Input: part model. Units: mm. Frame: model coordinates. Coordinates: 2 decimals unless noted, no trailing zeros. Order: outer loops, then holes, each group sorted by start corner. A loop starts at its lowest first (then second) coordinate and runs counter-clockwise, first axis right, second up. Notation, with made-up numbers: M -3.75,25.5 L 36.25,25.5 A20 cw 36.25,40.5 Z; hole C -10.5,9 d9. An arc over 180 degrees is marked long. One line per item, written item: value.
```python
from build123d import *

# Parameters (mm, degrees)
SKETCH2_W                = 22
SKETCH2_H                = 5
BOSS_EXTRUDE2_DEPTH      = 7.5
SKETCH16_W               = 0.596885676
SKETCH16_H               = 0.19726192
BOSS_EXTRUDE6_DEPTH      = 0.5
SKETCH17_W               = 0.596885676
SKETCH17_H               = 0.196118077
BOSS_EXTRUDE7_DEPTH      = 7.4
LPATTERN2_COUNT          = 10
LPATTERN2_PITCH          = 2.2
MIRROR1_COPY_1_SKETCH_W  = 0.596885676
MIRROR1_COPY_1_SKETCH_H  = 0.19726192
MIRROR1_COPY_1_DEPTH     = 0.5
MIRROR1_COPY_2_SKETCH_W  = 0.596885676
MIRROR1_COPY_2_SKETCH_H  = 0.19726192
MIRROR1_COPY_2_DEPTH     = 0.5
MIRROR1_COPY_3_SKETCH_W  = 0.596885676
MIRROR1_COPY_3_SKETCH_H  = 0.19726192
MIRROR1_COPY_3_DEPTH     = 0.5
MIRROR1_COPY_4_SKETCH_W  = 0.596885676
MIRROR1_COPY_4_SKETCH_H  = 0.19726192
MIRROR1_COPY_4_DEPTH     = 0.5
MIRROR1_COPY_5_SKETCH_W  = 0.596885676
MIRROR1_COPY_5_SKETCH_H  = 0.19726192
MIRROR1_COPY_5_DEPTH     = 0.5
MIRROR1_COPY_6_SKETCH_W  = 0.596885676
MIRROR1_COPY_6_SKETCH_H  = 0.19726192
MIRROR1_COPY_6_DEPTH     = 0.5
MIRROR1_COPY_7_SKETCH_W  = 0.596885676
MIRROR1_COPY_7_SKETCH_H  = 0.19726192
MIRROR1_COPY_7_DEPTH     = 0.5
MIRROR1_COPY_8_SKETCH_W  = 0.596885676
MIRROR1_COPY_8_SKETCH_H  = 0.19726192
MIRROR1_COPY_8_DEPTH     = 0.5
MIRROR1_COPY_9_SKETCH_W  = 0.596885676
MIRROR1_COPY_9_SKETCH_H  = 0.19726192
MIRROR1_COPY_9_DEPTH     = 0.5
MIRROR1_COPY_10_SKETCH_W = 0.596885676
MIRROR1_COPY_10_SKETCH_H = 0.196118077
MIRROR1_COPY_10_DEPTH    = 7.4
MIRROR1_COPY_11_SKETCH_W = 0.596885676
MIRROR1_COPY_11_SKETCH_H = 0.196118077
MIRROR1_COPY_11_DEPTH    = 7.4
MIRROR1_COPY_12_SKETCH_W = 0.596885676
MIRROR1_COPY_12_SKETCH_H = 0.196118077
MIRROR1_COPY_12_DEPTH    = 7.4
MIRROR1_COPY_13_SKETCH_W = 0.596885676
MIRROR1_COPY_13_SKETCH_H = 0.196118077
MIRROR1_COPY_13_DEPTH    = 7.4
MIRROR1_COPY_14_SKETCH_W = 0.596885676
MIRROR1_COPY_14_SKETCH_H = 0.196118077
MIRROR1_COPY_14_DEPTH    = 7.4
MIRROR1_COPY_15_SKETCH_W = 0.596885676
MIRROR1_COPY_15_SKETCH_H = 0.196118077
MIRROR1_COPY_15_DEPTH    = 7.4
MIRROR1_COPY_16_SKETCH_W = 0.596885676
MIRROR1_COPY_16_SKETCH_H = 0.196118077
MIRROR1_COPY_16_DEPTH    = 7.4
MIRROR1_COPY_17_SKETCH_W = 0.596885676
MIRROR1_COPY_17_SKETCH_H = 0.196118077
MIRROR1_COPY_17_DEPTH    = 7.4
MIRROR1_COPY_18_SKETCH_W = 0.596885676
MIRROR1_COPY_18_SKETCH_H = 0.196118077
MIRROR1_COPY_18_DEPTH    = 7.4


with BuildPart() as part:
    # Sketch2 → Boss-Extrude2 (new body)
    with BuildSketch(Plane(origin=(0, 5.922936542, 0), x_dir=(1, 0, 0), z_dir=(0, 0, 1))):
        with Locations((11, 2.5)):
            Rectangle(SKETCH2_W, SKETCH2_H)
    extrude(amount=BOSS_EXTRUDE2_DEPTH)

    # Sketch16 → Boss-Extrude6 (add)
    with BuildSketch(Plane.XY):
        with Locations((21, 8.422)):
            Rectangle(SKETCH16_W, SKETCH16_H)
    boss_extrude6 = extrude(amount=-BOSS_EXTRUDE6_DEPTH)

    # Sketch17 → Boss-Extrude7 (add)
    with BuildSketch(Plane.XZ.offset(-8.32336904)):
        with Locations((21, -0.401940962)):
            Rectangle(SKETCH17_W, SKETCH17_H)
    boss_extrude7 = extrude(amount=BOSS_EXTRUDE7_DEPTH)

    # LPattern2: Boss-Extrude6, Boss-Extrude7 ×10
    with Locations(*[(-i * LPATTERN2_PITCH, 0, 0) for i in range(1, LPATTERN2_COUNT)]):
        add(boss_extrude6)
        add(boss_extrude7)

    # Mirror1: Boss-Extrude6, Boss-Extrude7 across plane
    add(boss_extrude6.mirror(Plane(origin=(0, 0, 3.75), x_dir=(1, 0, 0), z_dir=(0, 0, -1))))
    add(boss_extrude7.mirror(Plane(origin=(0, 0, 3.75), x_dir=(1, 0, 0), z_dir=(0, 0, -1))))

    # Mirror1 copy 1 sketch → Mirror1 copy 1 (add)
    with BuildSketch(Plane(origin=(-2.2, 0, 7.5), x_dir=(1, 0, 0), z_dir=(0, 0, -1))):
        with Locations((21, -8.422)):
            Rectangle(MIRROR1_COPY_1_SKETCH_W, MIRROR1_COPY_1_SKETCH_H)
    extrude(amount=-MIRROR1_COPY_1_DEPTH)

    # Mirror1 copy 2 sketch → Mirror1 copy 2 (add)
    with BuildSketch(Plane(origin=(-4.4, 0, 7.5), x_dir=(1, 0, 0), z_dir=(0, 0, -1))):
        with Locations((21, -8.422)):
            Rectangle(MIRROR1_COPY_2_SKETCH_W, MIRROR1_COPY_2_SKETCH_H)
    extrude(amount=-MIRROR1_COPY_2_DEPTH)

    # Mirror1 copy 3 sketch → Mirror1 copy 3 (add)
    with BuildSketch(Plane(origin=(-6.6, 0, 7.5), x_dir=(1, 0, 0), z_dir=(0, 0, -1))):
        with Locations((21, -8.422)):
            Rectangle(MIRROR1_COPY_3_SKETCH_W, MIRROR1_COPY_3_SKETCH_H)
    extrude(amount=-MIRROR1_COPY_3_DEPTH)

    # Mirror1 copy 4 sketch → Mirror1 copy 4 (add)
    with BuildSketch(Plane(origin=(-8.8, 0, 7.5), x_dir=(1, 0, 0), z_dir=(0, 0, -1))):
        with Locations((21, -8.422)):
            Rectangle(MIRROR1_COPY_4_SKETCH_W, MIRROR1_COPY_4_SKETCH_H)
    extrude(amount=-MIRROR1_COPY_4_DEPTH)

    # Mirror1 copy 5 sketch → Mirror1 copy 5 (add)
    with BuildSketch(Plane(origin=(-11, 0, 7.5), x_dir=(1, 0, 0), z_dir=(0, 0, -1))):
        with Locations((21, -8.422)):
            Rectangle(MIRROR1_COPY_5_SKETCH_W, MIRROR1_COPY_5_SKETCH_H)
    extrude(amount=-MIRROR1_COPY_5_DEPTH)

    # Mirror1 copy 6 sketch → Mirror1 copy 6 (add)
    with BuildSketch(Plane(origin=(-13.2, 0, 7.5), x_dir=(1, 0, 0), z_dir=(0, 0, -1))):
        with Locations((21, -8.422)):
            Rectangle(MIRROR1_COPY_6_SKETCH_W, MIRROR1_COPY_6_SKETCH_H)
    extrude(amount=-MIRROR1_COPY_6_DEPTH)

    # Mirror1 copy 7 sketch → Mirror1 copy 7 (add)
    with BuildSketch(Plane(origin=(-15.4, 0, 7.5), x_dir=(1, 0, 0), z_dir=(0, 0, -1))):
        with Locations((21, -8.422)):
            Rectangle(MIRROR1_COPY_7_SKETCH_W, MIRROR1_COPY_7_SKETCH_H)
    extrude(amount=-MIRROR1_COPY_7_DEPTH)

    # Mirror1 copy 8 sketch → Mirror1 copy 8 (add)
    with BuildSketch(Plane(origin=(-17.6, 0, 7.5), x_dir=(1, 0, 0), z_dir=(0, 0, -1))):
        with Locations((21, -8.422)):
            Rectangle(MIRROR1_COPY_8_SKETCH_W, MIRROR1_COPY_8_SKETCH_H)
    extrude(amount=-MIRROR1_COPY_8_DEPTH)

    # Mirror1 copy 9 sketch → Mirror1 copy 9 (add)
    with BuildSketch(Plane(origin=(-19.8, 0, 7.5), x_dir=(1, 0, 0), z_dir=(0, 0, -1))):
        with Locations((21, -8.422)):
            Rectangle(MIRROR1_COPY_9_SKETCH_W, MIRROR1_COPY_9_SKETCH_H)
    extrude(amount=-MIRROR1_COPY_9_DEPTH)

    # Mirror1 copy 10 sketch → Mirror1 copy 10 (add)
    with BuildSketch(Plane(origin=(-2.2, 8.32336904, 7.5), x_dir=(1, 0, 0), z_dir=(0, -1, 0))):
        with Locations((21, 0.401940962)):
            Rectangle(MIRROR1_COPY_10_SKETCH_W, MIRROR1_COPY_10_SKETCH_H)
    extrude(amount=MIRROR1_COPY_10_DEPTH)

    # Mirror1 copy 11 sketch → Mirror1 copy 11 (add)
    with BuildSketch(Plane(origin=(-4.4, 8.32336904, 7.5), x_dir=(1, 0, 0), z_dir=(0, -1, 0))):
        with Locations((21, 0.401940962)):
            Rectangle(MIRROR1_COPY_11_SKETCH_W, MIRROR1_COPY_11_SKETCH_H)
    extrude(amount=MIRROR1_COPY_11_DEPTH)

    # Mirror1 copy 12 sketch → Mirror1 copy 12 (add)
    with BuildSketch(Plane(origin=(-6.6, 8.32336904, 7.5), x_dir=(1, 0, 0), z_dir=(0, -1, 0))):
        with Locations((21, 0.401940962)):
            Rectangle(MIRROR1_COPY_12_SKETCH_W, MIRROR1_COPY_12_SKETCH_H)
    extrude(amount=MIRROR1_COPY_12_DEPTH)

    # Mirror1 copy 13 sketch → Mirror1 copy 13 (add)
    with BuildSketch(Plane(origin=(-8.8, 8.32336904, 7.5), x_dir=(1, 0, 0), z_dir=(0, -1, 0))):
        with Locations((21, 0.401940962)):
            Rectangle(MIRROR1_COPY_13_SKETCH_W, MIRROR1_COPY_13_SKETCH_H)
    extrude(amount=MIRROR1_COPY_13_DEPTH)

    # Mirror1 copy 14 sketch → Mirror1 copy 14 (add)
    with BuildSketch(Plane(origin=(-11, 8.32336904, 7.5), x_dir=(1, 0, 0), z_dir=(0, -1, 0))):
        with Locations((21, 0.401940962)):
            Rectangle(MIRROR1_COPY_14_SKETCH_W, MIRROR1_COPY_14_SKETCH_H)
    extrude(amount=MIRROR1_COPY_14_DEPTH)

    # Mirror1 copy 15 sketch → Mirror1 copy 15 (add)
    with BuildSketch(Plane(origin=(-13.2, 8.32336904, 7.5), x_dir=(1, 0, 0), z_dir=(0, -1, 0))):
        with Locations((21, 0.401940962)):
            Rectangle(MIRROR1_COPY_15_SKETCH_W, MIRROR1_COPY_15_SKETCH_H)
    extrude(amount=MIRROR1_COPY_15_DEPTH)

    # Mirror1 copy 16 sketch → Mirror1 copy 16 (add)
    with BuildSketch(Plane(origin=(-15.4, 8.32336904, 7.5), x_dir=(1, 0, 0), z_dir=(0, -1, 0))):
        with Locations((21, 0.401940962)):
            Rectangle(MIRROR1_COPY_16_SKETCH_W, MIRROR1_COPY_16_SKETCH_H)
    extrude(amount=MIRROR1_COPY_16_DEPTH)

    # Mirror1 copy 17 sketch → Mirror1 copy 17 (add)
    with BuildSketch(Plane(origin=(-17.6, 8.32336904, 7.5), x_dir=(1, 0, 0), z_dir=(0, -1, 0))):
        with Locations((21, 0.401940962)):
            Rectangle(MIRROR1_COPY_17_SKETCH_W, MIRROR1_COPY_17_SKETCH_H)
    extrude(amount=MIRROR1_COPY_17_DEPTH)

    # Mirror1 copy 18 sketch → Mirror1 copy 18 (add)
    with BuildSketch(Plane(origin=(-19.8, 8.32336904, 7.5), x_dir=(1, 0, 0), z_dir=(0, -1, 0))):
        with Locations((21, 0.401940962)):
            Rectangle(MIRROR1_COPY_18_SKETCH_W, MIRROR1_COPY_18_SKETCH_H)
    extrude(amount=MIRROR1_COPY_18_DEPTH)


solid = part.part
```
(1) Draft query along Z for faces 1 (the flat face through (0, 8, 4)), 2 (the flat face through (11, 5.923, 4)). Return one class per face: released by +Z, released by -Z, zero draft, split by the parting line, or undercut.
Data:
face 1: zero draft
face 2: undercut
(2) First-contact query: pin 1 (0.6 mm diameter, centred on x = 14.5, z = -0.5, fed in from +Y); pin 2 (4 mm diameter, centred on y = 2, z = 5, fed in from +X); pin 3 (0.6 mm diameter, centred on y = 5, z = -0.5, fed in from +X). Flat tips, straight axial feed; report the tip coordinate or a pass-through.
Data:
pin 1: stops at y = 8.52
pin 2: passes through
pin 3: stops at x = 21.3
(3) Cut plane B-B on x = 11. Output: boundary loops of the cut face in (y, z).
Data:
outline: M 5.92,0 L 10.92,0 L 10.92,7.5 L 5.92,7.5 Z
(4) Cut plane D-D on z = 0.5. Output: boundary loops of the cut face in (x, y).
Data:
outline: M 0,5.92 L 22,5.92 L 22,10.92 L 0,10.92 Z
(5) Cut plane A-A on y = 6.25. Give the number of separate pieces and of enclosed holes in the cut face, plus the area to 3 significant figures.
Data:
separate pieces: 21
enclosed holes: 0
area: 167 mm2
(6) Ray query, line 1 (Z direction, x = 14.5, y = 4.25); line 2 (Z direction, x = 21, y = 7); line 3 (Z direction, x = 11.5, y = 7). Return the intervals inside material, ascending. Write a range as from..to.
Data:
line 1: z = -0.5..-0.3, 7.8..8
line 2: z = -0.5..-0.3, 0..7.5, 7.8..8
line 3: z = 0..7.5
